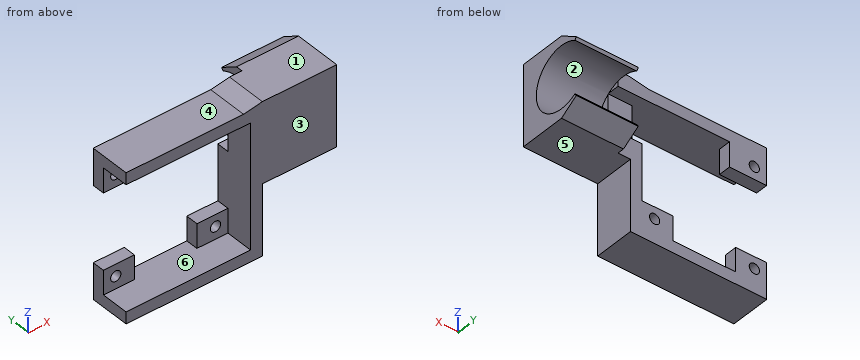
```python
from build123d import *

# Parameters (mm, degrees)
BOSS_EXTRUDE1_DEPTH = 9
SKETCH11_W          = 26
SKETCH11_H          = 9
BOSS_EXTRUDE2_DEPTH = 4
BOSS_EXTRUDE3_START = 4
BOSS_EXTRUDE3_DEPTH = 20
BOSS_EXTRUDE4_DEPTH = 9
SKETCH13_W          = 12
SKETCH13_H          = 8
SKETCH13_R          = 1.65
SKETCH13_H_2        = 3.8
SKETCH13_W_2        = 20.2
SKETCH13_W_3        = 4
SKETCH13_H_3        = 6.75
BOSS_EXTRUDE5_DEPTH = 4


with BuildPart() as part:
    # Sketch1 → Boss-Extrude1 (new body)
    with BuildSketch(Plane(origin=(0, 0, 0), x_dir=(1, 0, 0), z_dir=(0, 1, 0))):
        Polygon((-20.1, 20.1), (20.1, 20.1), (20.1, -20.1), (-20.1, -20.1), (-20.1, -23.9), (23.9, -23.9), (23.9, 23.9), (-20.1, 23.9), align=None)
    extrude(amount=BOSS_EXTRUDE1_DEPTH)

    # Sketch11 → Boss-Extrude2 (add)
    with BuildSketch(Plane(origin=(23.9, 0, 0), x_dir=(0, 0, -1), z_dir=(1, 0, 0))):
        with Locations((-11.95, 4.5)):
            Rectangle(SKETCH11_W, SKETCH11_H)
    extrude(amount=BOSS_EXTRUDE2_DEPTH)

    # Sketch10 → Boss-Extrude3 (add)
    with BuildSketch(Plane(origin=(23.9, 0, 0), x_dir=(0, 0, -1), z_dir=(1, 0, 0)).offset(BOSS_EXTRUDE3_START)):
        with BuildLine():
            Line((-21.257692308, 21.01232581), (-24.95, 15.15))
            Line((-24.95, 15.15), (-24.95, 0))
            Line((-24.95, 0), (1.05, 0))
            Line((1.05, 0), (1.05, 15.15))
            Line((1.05, 15.15), (-2.642307692, 21.01232581))
            Line((-2.642307692, 21.01232581), (-3.488461538, 20.4793871))
            ThreePointArc((-3.488461538, 20.4793871), (-11.95, 5.15), (-20.411538462, 20.4793871))
            Line((-20.411538462, 20.4793871), (-21.257692308, 21.01232581))
        make_face()
    extrude(amount=BOSS_EXTRUDE3_DEPTH)

    # Sketch12 → Boss-Extrude4 (add)
    with BuildSketch(Plane(origin=(0, 9, 0), x_dir=(1, 0, 0), z_dir=(0, 1, 0))):
        Polygon((23.9, -24.95), (17.829406445, -23.9), (23.9, -23.9), align=None)
    extrude(amount=-BOSS_EXTRUDE4_DEPTH)

    # Sketch13 → Boss-Extrude5 (add)
    # profile 1 of 9: a face of its own
    with BuildSketch(Plane(origin=(0, 9, 0), x_dir=(1, 0, 0), z_dir=(0, 1, 0))):
        with Locations((-14.1, -16.1)):
            Rectangle(SKETCH13_W, SKETCH13_H)
        with Locations(Location((-16.1, -16.1, 0), (0, 0, 270))):
            Circle(SKETCH13_R, mode=Mode.SUBTRACT)
    # profile 2 of 9: a face of its own
    with BuildSketch(Plane(origin=(0, 9, 0), x_dir=(1, 0, 0), z_dir=(0, 1, 0))):
        with Locations((-14.1, -22)):
            Rectangle(SKETCH13_W, SKETCH13_H_2)
    # profile 3 of 9: a face of its own
    with BuildSketch(Plane(origin=(0, 9, 0), x_dir=(1, 0, 0), z_dir=(0, 1, 0))):
        Polygon((27.9, -20.1), (-8.1, -20.1), (-8.1, -23.9), (17.829406445, -23.9), (27.9, -23.9), align=None)
    # profile 4 of 9: a face of its own
    with BuildSketch(Plane(origin=(0, 9, 0), x_dir=(1, 0, 0), z_dir=(0, 1, 0))):
        Polygon((27.9, -23.9), (17.829406445, -23.9), (23.9, -24.95), (27.9, -24.95), align=None)
    # profile 5 of 9: a face of its own
    with BuildSketch(Plane(origin=(0, 9, 0), x_dir=(1, 0, 0), z_dir=(0, 1, 0))):
        Polygon((23.9, 12.3), (23.9, 23.9), (10.1, 23.9), (10.1, 20.1), (10.1, 12.3), (20.1, 12.3), align=None)
        with Locations(Location((16.1, 16.1, 0), (0, 0, 270))):
            Circle(SKETCH13_R, mode=Mode.SUBTRACT)
    # profile 6 of 9: a face of its own
    with BuildSketch(Plane(origin=(0, 9, 0), x_dir=(1, 0, 0), z_dir=(0, 1, 0))):
        with Locations((0, 22)):
            Rectangle(SKETCH13_W_2, SKETCH13_H_2)
    # profile 7 of 9: a face of its own
    with BuildSketch(Plane(origin=(0, 9, 0), x_dir=(1, 0, 0), z_dir=(0, 1, 0))):
        Polygon((23.9, 1.05), (23.9, 12.3), (20.1, 12.3), (20.1, -5.7), (23.9, -5.7), align=None)
    # profile 8 of 9: a face of its own
    with BuildSketch(Plane(origin=(0, 9, 0), x_dir=(1, 0, 0), z_dir=(0, 1, 0))):
        Polygon((-10.1, 20.1), (-10.1, 23.9), (-20.1, 23.9), (-20.1, 12.3), (-10.1, 12.3), align=None)
        with Locations(Location((-16.1, 16.1, 0), (0, 0, 270))):
            Circle(SKETCH13_R, mode=Mode.SUBTRACT)
    # profile 9 of 9: a face of its own
    with BuildSketch(Plane(origin=(0, 9, 0), x_dir=(1, 0, 0), z_dir=(0, 1, 0))):
        with Locations((25.9, -2.325)):
            Rectangle(SKETCH13_W_3, SKETCH13_H_3)
    extrude(amount=BOSS_EXTRUDE5_DEPTH)


solid = part.part
```
Geometry: final body of the model. Coordinates: model frame, mm. Face numbers are marked on the shaded views. A direction names the side the tool comes from. Round coordinates to 2 decimals unless told otherwise and drop trailing zeros. Order: outer loops, then holes, each group sorted by start corner. A loop starts at its lowest first (then second) coordinate and runs counter-clockwise, first axis right, second up. Notation, with made-up numbers: (-2.5, -18.5) - (15.5, -18.5) arc R31 cw to (15.5, 7.5) - close; hole circle Ø7 at (36.5, 80). An arc over 180 degrees is marked (long way). Use CSV: the item, a comma, the result in double quotes. Start each with the question number.
Q1. Section query A-A (x = -16.1). Return loops of the section in (y, z), and give its area (3 significant figures).
Q2. Section query B-B (z = -16.5). Return loops of the section in (x, y).
Q3. Section query D-D (z = 13.5). Return loops of the section in (x, y).
Q4. Material intervals for line 1 along X through (y, z) = (11.1, -16.1); line 2 along X through (y, z) = (11.9, 16.1); line 3 along Z through (x, y) = (37.5, 15.15), sorted ascending. Write a range as from..to.
Q5. First-contact query: pin 1 (3 mm diameter, centred on x = -10, z = -16.5, fed in from +Y); pin 2 (1 mm diameter, centred on x = -10, y = 3.5, fed in from +Z); pin 3 (3 mm diameter, centred on x = 25.5, z = -17, fed in from +Y); pin 4 (8.5 mm diameter, centred on x = 16.5, z = -16.5, fed in from -Y). Flat tips, straight axial feed; report the tip coordinate or a pass-through.
Q6. Access query for the marked faces 4, 5 and 6. Directions: +Z, -Z, +X, -X, +Y, -Y. A direction counts if a zero-diameter tool reaches every point of the face in a straight line with its end or side. Return the directions, or none.
Q7. Mould query, pull axis Z, two halves, no side actions, for the marked faces 1, 2 and 3. Classes: +Z half, -Z half, draft (parallel to the pull), parting line (faces both ways), or undercut.
Q8. Section query C-C (x = 8). Return loops of the section in (y, z), and give its area (3 significant figures).
Result set:
1,outline,"(0, -23.9) - (13, -23.9) - (13, -17.75) - (9, -17.75) - (9, -20.1) - (0, -20.1) - close; (0, 20.1) - (9, 20.1) - (9, 17.75) - (13, 17.75) - (13, 23.9) - (0, 23.9) - close; (9, -14.45) - (13, -14.45) - (13, -12.3) - (9, -12.3) - close; (9, 12.1) - (13, 12.1) - (13, 14.45) - (9, 14.45) - close"
1,area,"136 mm2"
2,outline,"(-20.1, 9) - (-17.7, 9) - (-17.7, 13) - (-20.1, 13) - close; (-14.5, 9) - (-10.1, 9) - (-10.1, 13) - (-14.5, 13) - close; (10.1, 9) - (14.5, 9) - (14.5, 13) - (10.1, 13) - close; (17.7, 9) - (20.1, 9) - (20.1, 0) - (23.9, 0) - (23.9, 13) - (17.7, 13) - close"
3,outline,"(-20.1, 9) - (-8.1, 9) - (-8.1, 13) - (-20.1, 13) - close; (20.1, 0) - (47.9, 0) - (47.9, 5.27) - (27.9, 5.27) - (27.9, 9) - (20.1, 9) - close"
4,line 1,"x = -20.1..-17.75, -14.45..-10.1, 10.1..14.45, 17.75..23.9"
4,line 2,"x = -20.1..-17.75, -14.45..-8.1"
4,line 3,"z = -1.05..1.95, 21.95..24.95"
5,pin 1,"stops at y = 13"
5,pin 2,"stops at z = 23.9"
5,pin 3,"passes through"
5,pin 4,"stops at y = 0"
6,face 4,"+Z, -X, +Y, -Y"
6,face 5,"-Z, +X, +Y, -Y"
6,face 6,"-Y"
7,face 1,"+Z half"
7,face 2,"undercut"
7,face 3,"draft"
8,outline,"(0, -23.9) - (13, -23.9) - (13, -20.1) - (0, -20.1) - close; (0, 20.1) - (13, 20.1) - (13, 23.9) - (0, 23.9) - close"
8,area,"98.8 mm2"
